Could you check a few things on this drawing? It's one solid part, dimensions in mm from its lowest x, y, z. Coordinates: 2 decimals unless noted, no trailing zeros. Order: outer loops, then holes, each group sorted by start corner. A loop starts at its lowest first (then second) coordinate and runs counter-clockwise, first axis right, second up.
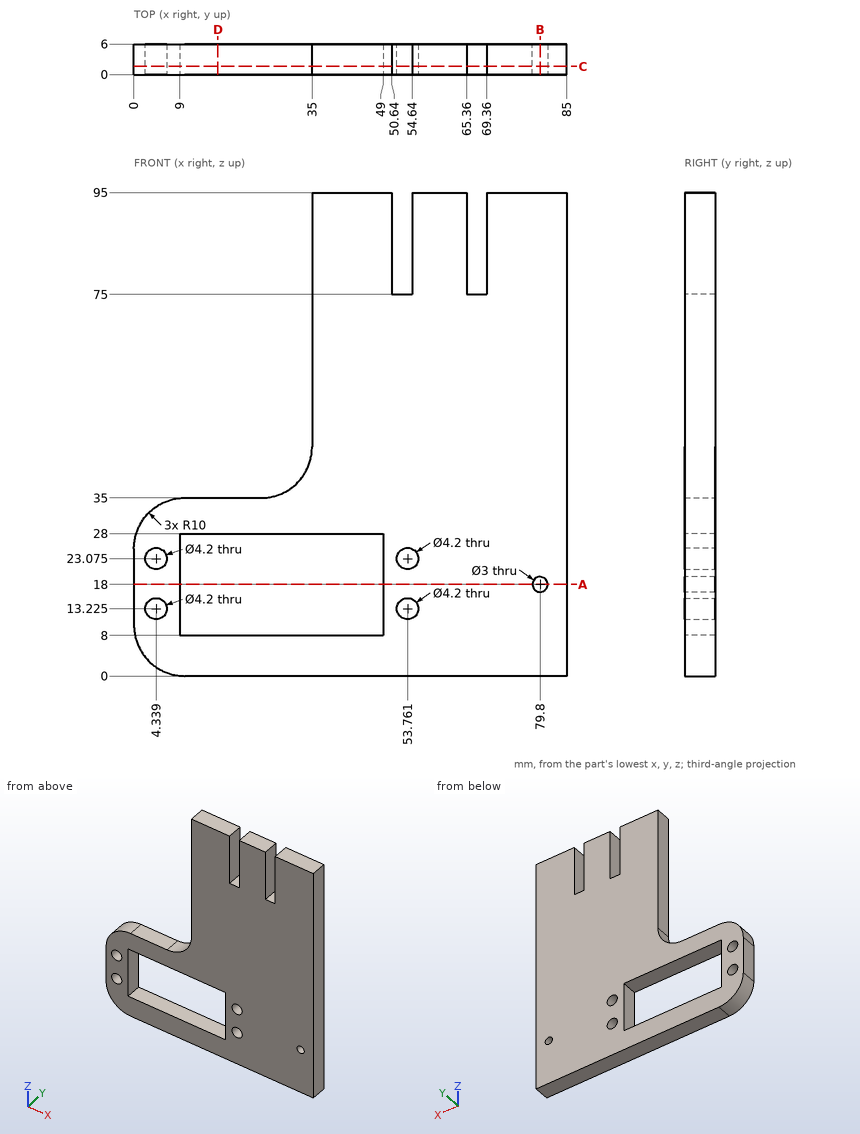
1. Imagine slicing it at B-B on x = 79.8. Please give me the cut outline in (y, z).
Completed:
outline: (0, 0) - (6, 0) - (6, 16.5) - (0, 16.5) - close; (0, 19.5) - (6, 19.5) - (6, 95) - (0, 95) - close
2. I'm going to push a flat-ended pin straight in: pin 1 (3 mm diameter, centred on y = 2, z = 59.5, fed in from -X). Where does the tip first touch, or does it pass through?
Completed:
pin 1: stops at x = 35
3. Imagine slicing it at D-D on x = 16.5. Please give me the cut outline in (y, z).
Completed:
outline: (0, 0) - (6, 0) - (6, 8) - (0, 8) - close; (0, 28) - (6, 28) - (6, 35) - (0, 35) - close
4. Please list where these lines run through material, in increasing order: probe 1 along Z at (x, y) = (53.5, 1.55); probe 2 along Z at (x, y) = (79.8, 3.3); probe 3 along X at (y, z) = (2.9, 77.5).
Completed:
probe 1: z = 0 to 11.14, 15.31 to 20.99, 25.16 to 75
probe 2: z = 0 to 16.5, 19.5 to 95
probe 3: x = 35 to 50.64, 54.64 to 65.36, 69.36 to 85
5. Imagine slicing it at A-A on z = 18. Please give me the cut outline in (x, y).
Completed:
outline: (0, 0) - (9, 0) - (9, 6) - (0, 6) - close; (49, 0) - (78.3, 0) - (78.3, 6) - (49, 6) - close; (81.3, 0) - (85, 0) - (85, 6) - (81.3, 6) - close
6. Imagine slicing it at C-C on y = 1.6. Please give me the cut outline in (x, z) (3 decimals).
Completed:
outline: (0, 10) arc R10 ccw to (10, 0) - (85, 0) - (85, 95) - (69.36, 95) - (69.36, 75) - (65.36, 75) - (65.36, 95) - (54.64, 95) - (54.64, 75) - (50.64, 75) - (50.64, 95) - (35, 95) - (35, 45) arc R10 cw to (25, 35) - (10, 35) arc R10 ccw to (0, 25) - close; hole circle Ø4.2 at (4.339, 13.225); hole circle Ø4.2 at (4.339, 23.075); hole (9, 8) - (49, 8) - (49, 28) - (9, 28) - close; hole circle Ø4.2 at (53.761, 13.225); hole circle Ø4.2 at (53.761, 23.075); hole circle Ø3 at (79.8, 18)
